CAD build for the part. Positions are in the model's coordinates, mm. Face numbers are marked on the shaded views. Give positions to 0.01 mm unless a question says otherwise; leave off trailing zeros. Write each loop counter-clockwise with the first axis right and the second up, starting at its lowest first coordinate (ties: lowest second). Pieces come first, ordered by that corner, then holes. Notation, with made-up numbers: (-30.75, 52.5) -> (-21.75, 52.5) arc R26 cw to (-21.75, 72.5) -> close; hole circle Ø11 at (-19.75, 34). An arc over 180 degrees is marked (long way). Answer as a JSON object with one key per item and string values.
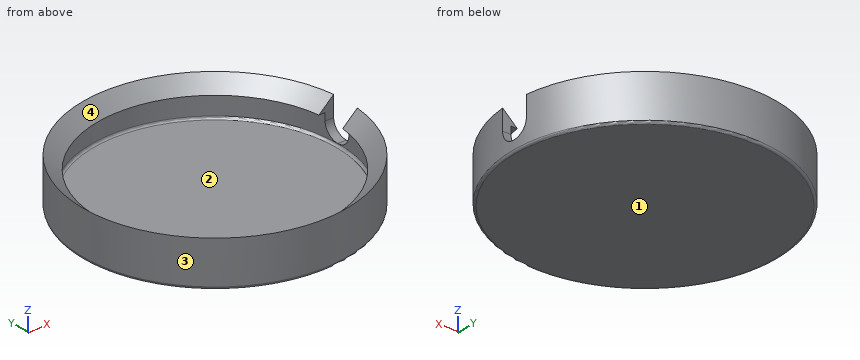
```python
from build123d import *

# Parameters (mm, degrees)
F0_R     = 29.718
F1_DEPTH = 10.16
F6_R     = 0.508
F8_W     = 4.7481491719
F8_H     = 6.35
F9_DEPTH = 25.4
F10_R    = 3.17499


# Not quite as in the source:
# - a fillet or chamfer is up to 0.001 mm smaller than in the source, because OpenCascade refuses the exact size


with BuildPart() as f1:
    # F0 (on Top) → F1 (new body)
    with BuildSketch(Plane.XY):
        Circle(F0_R)
    extrude(amount=F1_DEPTH)

    # F2 (on Front) → F3 (revolve, cut)
    with BuildSketch(Plane.XZ):
        Polygon((29.718, 10.16), (0, 10.16), (0, 7.2644), (26.416, 7.2644), align=None)
    revolve(axis=Axis((0, 0, 8.7122), (0, 0, 1)), mode=Mode.SUBTRACT)

    # F4 (on Front) → F5 (revolve, cut)
    with BuildSketch(Plane.XZ):
        Polygon((0, 7.2644), (-26.416, 7.2644), (-27.813, 7.2644), (-27.813, 1.905), (0, 1.905), align=None)
    revolve(axis=Axis((0, 0, 4.5847), (0, 0, 1)), mode=Mode.SUBTRACT)

    # F6
    f6_edges = [f1.edges().sort_by_distance(p)[0] for p in [
        (27.813, 0, 1.905),
        (-29.718, 0, 0),
    ]]
    fillet(f6_edges, radius=F6_R)

    # F8 (on face) → F9 (cut)
    with BuildSketch(Plane.XY.offset(2.413)):
        with Locations((28.1168716028, 0)):
            Rectangle(F8_W, F8_H)
    extrude(amount=F9_DEPTH, mode=Mode.SUBTRACT)

    # F10 (radius 3.175 in the source; OpenCascade refuses exactly that, so slightly less here)
    f10_edges = [f1.edges().sort_by_distance(p)[0] for p in [
        (28.589546, 3.175, 2.413),
        (28.589546, -3.175, 2.413),
    ]]
    fillet(f10_edges, radius=F10_R)


solid = f1.part
```
1) Pin check, flat tips, straight feed: pin 1 (1 mm diameter, centred on x = 28, z = 8, fed in from +Y); pin 2 (5 mm diameter, centred on x = 12.5, y = -11.5, fed in from +Z) (3 decimals); pin 3 (2 mm diameter, centred on y = -5.5, z = 6, fed in from -X). Stop position of each tip, or through.
Model answer:
{"pin 1": "stops at y = 11.27", "pin 2": "stops at z = 1.905", "pin 3": "stops at x = -29.38"}
2) Wall check: probe 1 along Y at (x, z) = (-0.5, 6.25); probe 2 along Y at (x, z) = (-16, 4); probe 3 along Z at (x, y) = (-15, 19.5) (3 decimals). Give the ranges that are in metal, low to high.
Model answer:
{"probe 1": "y = -29.71 to -27.81, 27.81 to 29.71", "probe 2": "y = -25.04 to -22.75, 22.75 to 25.04", "probe 3": "z = 0 to 1.905"}
3) Mould opens along Y. For the marked faces 1, 2, 3 and 4 say: released by +Y, released by -Y, zero draft, split by the parting line, or undercut.
Model answer:
{"face 1": "zero draft", "face 2": "undercut", "face 3": "split by the parting line", "face 4": "undercut"}
4) Slice it at B-B (z = 6.5). List the corners of the cut face in (x, y) (3 decimals).
Model answer:
{"outline": "(27.631, -3.175) arc R27.813 cw (long way) to (27.631, 3.175) -> (29.548, 3.175) arc R29.718 ccw (long way) to (29.548, -3.175) -> close"}
5) Slice it at A-A (x = 0). List the corners of the cut face in (y, z) (3 decimals), then the cut area to 3 significant figures.
Model answer:
{"outline": "(-29.718, 0.508) arc R0.508 ccw to (-29.21, 0) -> (29.21, 0) arc R0.508 ccw to (29.718, 0.508) -> (29.718, 10.16) -> (26.416, 7.264) -> (27.813, 7.264) -> (27.813, 2.413) arc R0.508 cw to (27.305, 1.905) -> (-27.305, 1.905) arc R0.508 cw to (-27.813, 2.413) -> (-27.813, 7.264) -> (-26.416, 7.264) -> (-29.718, 10.16) -> close", "area": "143 mm2"}
